```python
from build123d import *

# Parameters (mm, degrees)
SKETCH1_W           = 36
SKETCH1_H           = 40
BOSS_EXTRUDE1_DEPTH = 5
BOSS_EXTRUDE2_DEPTH = 5
BOSS_EXTRUDE4_DEPTH = 8
FILLET1_R           = 1
FILLET2_R           = 1
FILLET3_R           = 1
SKETCH4_R           = 1.9
CUT_EXTRUDE1_DEPTH  = 91.049986119
SKETCH5_R           = 2.5
BOSS_EXTRUDE5_DEPTH = 3.5
SKETCH6_R           = 1.45
CUT_EXTRUDE2_DEPTH  = 7
SKETCH7_W           = 36
SKETCH7_H           = 40
BOSS_EXTRUDE6_DEPTH = 30
SKETCH8_R           = 31.5
BOSS_EXTRUDE7_DEPTH = 8
SKETCH9_R           = 3.1
CUT_EXTRUDE3_DEPTH  = 8
FILLET5_R           = 1
FILLET6_R           = 1
SKETCH10_R          = 1.4
CUT_EXTRUDE4_DEPTH  = 10


with BuildPart() as part:
    # Sketch1 → Boss-Extrude1 (new body)
    with BuildSketch(Plane(origin=(0, 0, 0), x_dir=(1, 0, 0), z_dir=(0, 1, 0))):
        Rectangle(SKETCH1_W, SKETCH1_H)
    extrude(amount=BOSS_EXTRUDE1_DEPTH)

    # Sketch2 → Boss-Extrude2 (add)
    with BuildSketch(Plane(origin=(0, 5, 0), x_dir=(1, 0, 0), z_dir=(0, 1, 0))):
        Polygon((-18, -20), (-18, 62), (-26, 62), (-26, -28), (64, -28), (64, -20), align=None)
    extrude(amount=-BOSS_EXTRUDE2_DEPTH)

    # Sketch3 → Boss-Extrude4 (add)
    with BuildSketch(Plane(origin=(0, 5, 0), x_dir=(1, 0, 0), z_dir=(0, 1, 0))):
        with BuildLine():
            Line((-18, 20), (18, 20))
            Line((18, 20), (18, -20))
            Line((18, -20), (8, -20))
            Line((8, -20), (8, -18.2))
            Line((8, -18.2), (16.2, -18.2))
            Line((16.2, -18.2), (16.2, 18.2))
            Line((16.2, 18.2), (-16.2, 18.2))
            Line((-16.2, 18.2), (-16.2, -18.2))
            Line((-16.2, -18.2), (-8, -18.2))
            Line((-8, -18.2), (-8, -20))
            Line((-8, -20), (-16, -20))
            ThreePointArc((-16, -20), (-17.414213562, -20.585786438), (-18, -22))
            Line((-18, -22), (-18, -28))
            Line((-18, -28), (-26, -28))
            Line((-26, -28), (-26, -20))
            Line((-26, -20), (-20, -20))
            ThreePointArc((-20, -20), (-18.585786438, -19.414213562), (-18, -18))
            Line((-18, -18), (-18, 20))
        make_face()
    extrude(amount=BOSS_EXTRUDE4_DEPTH)

    # Fillet1
    # the kernel refuses this fillet: 1 mm, written as the material it adds along each edge
    with BuildSketch(Plane(origin=(16.2, 2.5, 18.2), x_dir=(0, 0, -1), z_dir=(0, 1, 0)), Plane(origin=(16.2, 2.5, -18.2), x_dir=(-1, 0, 0), z_dir=(0, 1, 0)), Plane(origin=(-16.2, 2.5, -18.2), x_dir=(0, 0, 1), z_dir=(0, 1, 0)), Plane(origin=(-16.2, 2.5, 18.2), x_dir=(1, 0, 0), z_dir=(0, 1, 0))) as fillet1_piece_1:
        with BuildLine():
            CenterArc((FILLET1_R, FILLET1_R), FILLET1_R, 180, 90)
            Line((0, FILLET1_R), (0, 0))
            Line((0, 0), (FILLET1_R, 0))
        make_face()
    extrude(amount=10.5)
    # the kernel refuses this fillet: 1 mm, written as the material it takes off along each edge
    with BuildSketch(Plane(origin=(-26, 15.5, 28), x_dir=(1, 0, 0), z_dir=(0, -1, 0))) as fillet1_2_piece_1:
        with BuildLine():
            CenterArc((FILLET1_R, -FILLET1_R), FILLET1_R, 90, 90)
            Line((0, -FILLET1_R), (0, 0))
            Line((0, 0), (FILLET1_R, 0))
        make_face()
    extrude(amount=18, mode=Mode.SUBTRACT)
    with BuildSketch(Plane(origin=(-26, 5, 20), x_dir=(0, 0, 1), z_dir=(0, 1, 0)), Plane(origin=(-18, 5, 28), x_dir=(0, 0, -1), z_dir=(0, 1, 0)), Plane(origin=(8, 5, 20), x_dir=(1, 0, 0), z_dir=(0, 1, 0)), Plane(origin=(8, 5, 18.2), x_dir=(0, 0, 1), z_dir=(0, 1, 0)), Plane(origin=(-8, 5, 18.2), x_dir=(-1, 0, 0), z_dir=(0, 1, 0)), Plane(origin=(-8, 5, 20), x_dir=(0, 0, -1), z_dir=(0, 1, 0))) as fillet1_2_piece_2:
        with BuildLine():
            CenterArc((FILLET1_R, FILLET1_R), FILLET1_R, 180, 90)
            Line((0, FILLET1_R), (0, 0))
            Line((0, 0), (FILLET1_R, 0))
        make_face()
    extrude(amount=10.5, mode=Mode.SUBTRACT)

    # Fillet2
    fillet2_edges = [part.edges().sort_by_distance(p)[0] for p in [
        (-18, 9, -20),
        (18, 9, 20),
    ]]
    fillet(fillet2_edges, radius=FILLET2_R)

    # Fillet3
    fillet3_edges = [part.edges().sort_by_distance(p)[0] for p in [
        (-18, 2.5, -62),
        (64, 2.5, 20),
        (64, 2.5, 28),
        (-26, 2.5, -62),
    ]]
    fillet(fillet3_edges, radius=FILLET3_R)

    # Sketch4 → Cut-Extrude1 (cut, through all)
    with BuildSketch(Plane(origin=(0, 13, 0), x_dir=(1, 0, 0), z_dir=(0, 1, 0))):
        with Locations(Location((-22, -24, 0), (0, 0, 270))):
            Circle(SKETCH4_R)
        with Locations(Location((-22, 51, 0), (0, 0, 270))):
            Circle(SKETCH4_R)
        with Locations(Location((60, -24, 0), (0, 0, 270))):
            Circle(SKETCH4_R)
    extrude(amount=-CUT_EXTRUDE1_DEPTH, mode=Mode.SUBTRACT)

    # Sketch5 → Boss-Extrude5 (add)
    with BuildSketch(Plane(origin=(0, 5, 0), x_dir=(1, 0, 0), z_dir=(0, 1, 0))):
        with Locations(Location((-11.425, 14, 0), (0, 0, 270))):
            Circle(SKETCH5_R)
        with Locations(Location((11.425, 14, 0), (0, 0, 270))):
            Circle(SKETCH5_R)
        with Locations(Location((11.425, -14, 0), (0, 0, 270))):
            Circle(SKETCH5_R)
        with Locations(Location((-11.425, -14, 0), (0, 0, 270))):
            Circle(SKETCH5_R)
    extrude(amount=BOSS_EXTRUDE5_DEPTH)

    # Sketch6 → Cut-Extrude2 (cut)
    with BuildSketch(Plane(origin=(0, 8.5, 0), x_dir=(1, 0, 0), z_dir=(0, 1, 0))):
        with Locations(Location((-11.425, 14, 0), (0, 0, 270))):
            Circle(SKETCH6_R)
        with Locations(Location((11.425, 14, 0), (0, 0, 270))):
            Circle(SKETCH6_R)
        with Locations(Location((11.425, -14, 0), (0, 0, 270))):
            Circle(SKETCH6_R)
        with Locations(Location((-11.425, -14, 0), (0, 0, 270))):
            Circle(SKETCH6_R)
    extrude(amount=-CUT_EXTRUDE2_DEPTH, mode=Mode.SUBTRACT)

    # Sketch7 → Boss-Extrude6 (add)
    with BuildSketch(Plane.XZ):
        Rectangle(SKETCH7_W, SKETCH7_H)
    extrude(amount=BOSS_EXTRUDE6_DEPTH)

    # Sketch8 → Boss-Extrude7 (add)
    with BuildSketch(Plane.XZ.offset(30)):
        with Locations(Location((0, 0, 0), (0, 0, 270))):
            Circle(SKETCH8_R)
    extrude(amount=BOSS_EXTRUDE7_DEPTH)

    # Sketch9 → Cut-Extrude3 (cut)
    with BuildSketch(Plane.XZ.offset(38)):
        with Locations(Location((0, 25, 0), (0, 0, 270))):
            Circle(SKETCH9_R)
        with Locations(Location((-25, 0, 0), (0, 0, 270))):
            Circle(SKETCH9_R)
        with Locations(Location((25, 0, 0), (0, 0, 270))):
            Circle(SKETCH9_R)
        with Locations(Location((0, -25, 0), (0, 0, 270))):
            Circle(SKETCH9_R)
    extrude(amount=-CUT_EXTRUDE3_DEPTH, mode=Mode.SUBTRACT)

    # Fillet5
    fillet5_edges = [part.edges().sort_by_distance(p)[0] for p in [
        (-18, -15, 20),
        (-18, -15, -20),
        (18, -15, 20),
        (18, -8.5, -20),
    ]]
    fillet(fillet5_edges, radius=FILLET5_R)

    # Fillet6
    fillet6_edges = [part.edges().sort_by_distance(p)[0] for p in [
        (-18, 2.5, -20),
        (18, 2.5, 20),
    ]]
    fillet(fillet6_edges, radius=FILLET6_R)

    # Sketch10 → Cut-Extrude4 (cut)
    with BuildSketch(Plane(origin=(18, 0, 0), x_dir=(0, 0, -1), z_dir=(1, 0, 0))):
        with Locations((-10, -12)):
            Circle(SKETCH10_R)
        with Locations((-10, 3)):
            Circle(SKETCH10_R)
    extrude(amount=-CUT_EXTRUDE4_DEPTH, mode=Mode.SUBTRACT)


solid = part.part
```
Source: CAD feature listing. Evaluate the final solid. Frame: model axes, mm. A direction names the side the tool comes from. Round coordinates to 2 decimals unless told otherwise and drop trailing zeros. Loops run counter-clockwise (first coordinate to the right, second up) from the corner with the lowest first, then second, coordinate; pieces in that order, holes last. Notation, with made-up numbers: M 2.5,37 L 45.5,37 A18 cw 45.5,62 Z; hole C 59,-28.5 d11. An arc over 180 degrees is marked long. Use a Markdown table: item, result. Add a question column.
1. Section query B-B on z = 24. Return the cut outline in (x, y), then the cut area to 3 significant figures.
2. Mould query, pull axis X, two halves, no side actions, for faces 1 (the cylindrical face through (10.14, 5.05, -13.33)), 2 (the flat face through (-18, 3, -41)), 3 (the flat face through (-18, 9, 0)). Classes: pulls with the +X half, pulls with the -X half, needs draft (parallel to the pull), parting line crosses it, or undercut.
3. Section query A-A on x = 0. Return the cut outline in (y, z), then the cut area to 3 significant figures.
4. Section query C-C on x = 60. Return the cut outline in (y, z).
5. Contact query for flat-ended pins moving along their axis: P1, Ø7, axis at x = -25, z = 0, coming from the -Y side; P2, Ø1.5, axis at x = -4, y = 2, coming from the +Z side; P3, Ø1.5, axis at y = -23, z = -2, coming from the -X side; P4, Ø5.5, axis at x = 11, z = 14, coming from the +Y side. Output: stop coordinate, or through.
6. Line query: line 1 (X direction, y = -36, z = 0); line 2 (Y direction, x = 13.5, z = 10); line 3 (Y direction, x = -25.5, z = 15). Output: solid intervals per line, ascending.
7. Reachability of faces 4 (the cylindrical face through (-10.202, 5.049, 14.78)), 5 (the flat face through (0, -15, 20)), 6 (the cylindrical face through (13.07, -11.05, 11.03)), 7 (the flat face through (13, 9, 20)) from +Z, -Z, +X, -X, +Y, -Y: full face, straight path, thin tool, end or side. Return the list, or none.
8. Section query D-D on z = -50.5. Return the cut outline in (x, y), then the cut area to 3 significant figures.
Reported:
| question | item | result |
|---|---|---|
| 1 | outline | M -26,0 L -23.9,0 L -23.9,13 L -26,13 Z; M -20.4,-38 L -2.93,-38 L -2.93,-30 L -20.4,-30 Z; M -20.1,0 L 58.1,0 L 58.1,5 L -18,5 L -18,13 L -20.1,13 Z; M 2.93,-38 L 20.4,-38 L 20.4,-30 L 2.93,-30 Z; M 61.9,0 L 64,0 L 64,5 L 61.9,5 Z |
| 1 | area | 725 mm² |
| 2 | face 1 | undercut |
| 2 | face 2 | pulls with the +X half |
| 2 | face 3 | pulls with the -X half |
| 3 | outline | M -38,-31.5 L -30,-31.5 L -30,-28.1 L -38,-28.1 Z; M -38,-21.9 L -30,-21.9 L -30,-20 L 13,-20 L 13,-18.2 L 5,-18.2 L 5,28 L 0,28 L 0,20 L -30,20 L -30,21.9 L -38,21.9 Z; M -38,28.1 L -30,28.1 L -30,31.5 L -38,31.5 Z |
| 3 | area | 1,860 mm² |
| 4 | outline | M 0,20 L 5,20 L 5,22.1 L 0,22.1 Z; M 0,25.9 L 5,25.9 L 5,28 L 0,28 Z |
| 5 | P1 | stops at y = -38 |
| 5 | P2 | stops at z = 28 |
| 5 | P3 | stops at x = -18 |
| 5 | P4 | stops at y = 8.5 |
| 6 | line 1 | x = -31.5 to -28.1, -21.9 to 21.9, 28.1 to 31.5 |
| 6 | line 2 | y = -38 to -13.4, -10.6 to 1.6, 4.4 to 5 |
| 6 | line 3 | y = -38 to -30, 0 to 5 |
| 7 | face 4 | +Y |
| 7 | face 5 | +Z, +X, -X |
| 7 | face 6 | +X |
| 7 | face 7 | +Z, +X, +Y |
| 8 | outline | M -26,0 L -23.83,0 L -23.83,5 L -26,5 Z; M -20.17,0 L -18,0 L -18,5 L -20.17,5 Z |
| 8 | area | 21.7 mm² |
